Geometry: see drawing. Coordinates: mm, zero at the bounding-box minimum. A direction names the side the tool comes from. Round coordinates to 2 decimals unless told otherwise and drop trailing zeros. Loops run counter-clockwise (first coordinate to the right, second up) from the corner with the lowest first, then second, coordinate; pieces in that order, holes last.
(1) Access query for the marked faces 5 and 6. Directions: +Z, -Z, +X, -X, +Y, -Y. A direction counts if a zero-diameter tool reaches every point of the face in a straight line with its end or side. Return the directions, or none.
(2) Cut plane C-C, the plane y = 9.25. Output: boundary loops of the cut face in (x, z).
(3) Cut plane A-A, the plane x = 30. Output: boundary loops of the cut face in (y, z) (1 decimal), and give its area (3 significant figures).
(4) Line query: line 1 (X direction, y = 5.75, z = 7); line 2 (Y direction, x = 56.5, z = 3.5) (3 decimals); line 3 (Y direction, x = 25.5, z = 2) (1 decimal). Output: solid intervals per line, ascending.
(5) First-contact query: pin 1 Ø10 at (x, y) = (29.38, 14.27) entering from -Z; pin 2 Ø5.5 at (x, z) = (56.5, 7) entering from +Y (3 decimals); pin 3 Ø6 at (y, z) = (11, 4.5) entering from -X; pin 4 Ø4 at (y, z) = (7, 5.5) entering from +X. Flat tips, straight axial feed; report the tip coordinate or a pass-through.
(6) Cut plane D-D, the plane y = 4.5. Output: boundary loops of the cut face in (x, z).
(7) Draft query along Y for the marked faces 1, 2, 3 and 4. Return one class per face: released by +Y, released by -Y, zero draft, split by the parting line, or undercut.
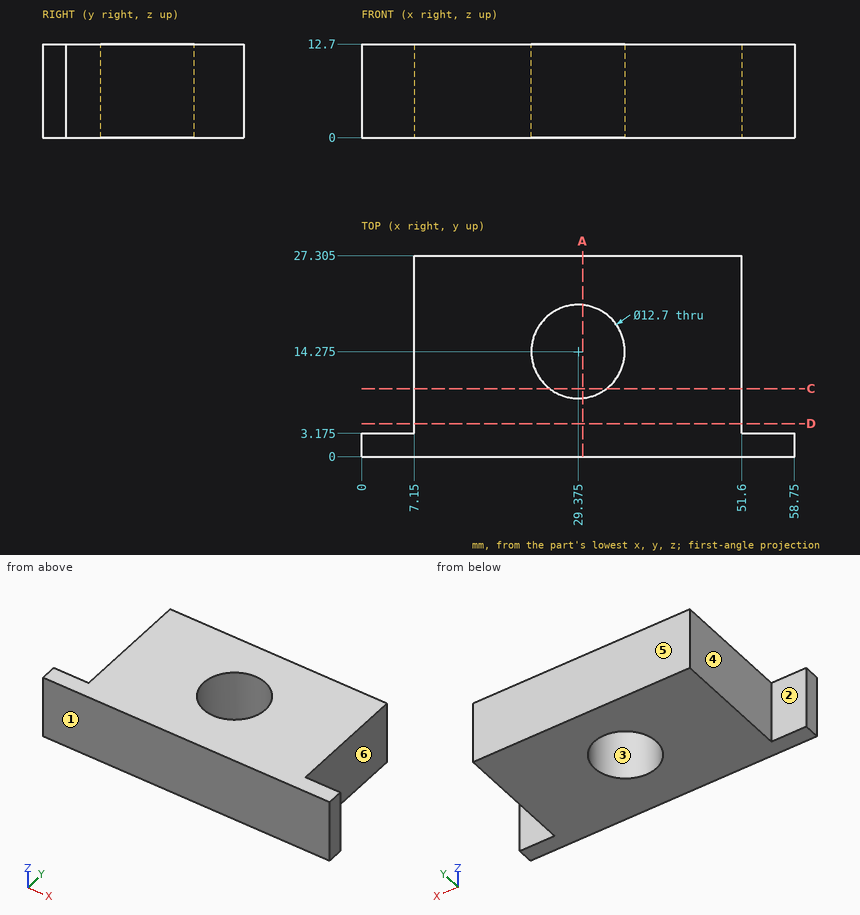
Reported:
1. face 5: +Z, -Z, +X, -X, +Y
1. face 6: +Z, -Z, +X, +Y
2. outline: (7.15, 0) - (25.49, 0) - (25.49, 12.7) - (7.15, 12.7) - close; (33.26, 0) - (51.6, 0) - (51.6, 12.7) - (33.26, 12.7) - close
3. outline: (0, 0) - (8, 0) - (8, 12.7) - (0, 12.7) - close; (20.6, 0) - (27.3, 0) - (27.3, 12.7) - (20.6, 12.7) - close
3. area: 186 mm2
4. line 1: x = 7.15 to 51.6
4. line 2: y = 0 to 3.175
4. line 3: y = 0 to 9.2, 19.3 to 27.3
5. pin 1: passes through
5. pin 2: stops at y = 3.175
5. pin 3: stops at x = 7.15
5. pin 4: stops at x = 51.6
6. outline: (7.15, 0) - (51.6, 0) - (51.6, 12.7) - (7.15, 12.7) - close
7. face 1: released by -Y
7. face 2: released by +Y
7. face 3: undercut
7. face 4: zero draft
